Part model, mm, in its own coordinate system. Face numbers are marked on the shaded views. A direction names the side the tool comes from. Round coordinates to 2 decimals unless told otherwise and drop trailing zeros. Order: outer loops, then holes, each group sorted by start corner. A loop starts at its lowest first (then second) coordinate and runs counter-clockwise, first axis right, second up. Notation, with made-up numbers: (29, 3.25) - (71, 3.25) arc R15 cw to (71, 17.25) - close; hole circle Ø5 at (29.25, 74). An arc over 180 degrees is marked (long way). Return JSON: item names as keys, results as strings. Group by question number.
Item 1: Saw through at A-A on y = 0. List the corners of the cut face in (x, z).
Item 2: Tool access for the marked faces 1 and 2: list every direction of +Z, -Z, +X, -X, +Y, -Y with a clear straight run to the whole face (end or side of a thin tool).
Item 3: Saw through at C-C on y = -11. List the corners of the cut face in (x, z).
Item 4: Drop flat-ended pins along their axis: pin 1 (6 mm diameter, centred on y = 11.5, z = 130.5, fed in from -X); pin 2 (15 mm diameter, centred on x = -7, y = 0, fed in from +Z); pin 3 (3 mm diameter, centred on x = 91, z = 134.5, fed in from +Y). Give the stop position or say it passes through.
Item 5: Probe probe 1 along X at (y, z) = (-4.5, 82.5); probe 2 along Z at (x, y) = (7, 6); probe 3 along Z at (x, y) = (157, 3). List the from-to ranges inside material, lowest first.
Item 6: Saw through at B-B on y = 9. List the corners of the cut face in (x, z), and give its area (3 significant figures).
Item 7: Two-plate mould, pull along X, no slides. Class the marked faces 3 and 4: released by +X, released by -X, zero draft, split by the parting line, or undercut.
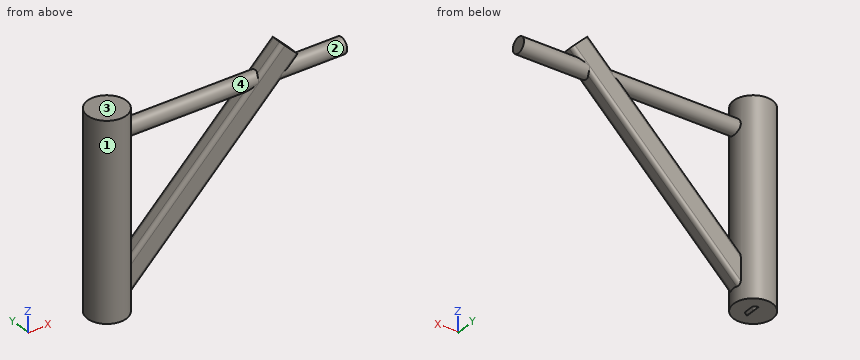
```python
from build123d import *

# Parameters (mm, degrees)
F0_R     = 15
F1_DEPTH = 150
F2_R     = 6
F3_DEPTH = 180
F7_DEPTH = 200


with BuildPart() as f1:
    # F0 (on Top) → F1 (new body)
    with BuildSketch(Plane.XY):
        Circle(F0_R)
    extrude(amount=F1_DEPTH)

    # F2 (on Right) → F3 (join)
    with BuildSketch(Plane.YZ):
        with Locations((0, 130.317822)):
            Circle(F2_R)
    extrude(amount=F3_DEPTH)

    # F6 (on face) → F7 (join)
    with BuildSketch(Plane(origin=(0, 0, 0), x_dir=(0.707107, 0, -0.707107), z_dir=(-0.707107, 0, -0.707107))):
        with BuildLine():
            Line((-0.517934, 6), (-12.829055, 6))
            ThreePointArc((-12.829055, 6), (-14.950375, 5.12132), (-15.829055, 3))
            Line((-15.829055, 3), (-15.829055, -3))
            ThreePointArc((-15.829055, -3), (-14.950375, -5.12132), (-12.829055, -6))
            Line((-12.829055, -6), (-0.517934, -6))
            ThreePointArc((-0.517934, -6), (1.603386, -5.12132), (2.482066, -3))
            Line((2.482066, -3), (2.482066, 3))
            ThreePointArc((2.482066, 3), (1.603386, 5.12132), (-0.517934, 6))
        make_face()
    extrude(amount=-F7_DEPTH)


solid = f1.part
```
Filled in:
{
 "1": {"outline": "(-15, 0) - (0, 0) - (1.76, -1.76) - (3.51, 0) - (15, 0) - (15, 11.49) - (127.83, 124.32) - (180, 124.32) - (180, 136.32) - (139.83, 136.32) - (143.18, 139.67) - (130.23, 152.61) - (113.93, 136.32) - (15, 136.32) - (15, 150) - (-15, 150) - close; hole (15, 37.39) - (101.93, 124.32) - (15, 124.32) - close"},
 "2": {"face 1": "none", "face 2": "+X"},
 "3": {"outline": "(-10.2, 0) - (10.2, 0) - (10.2, 150) - (-10.2, 150) - close"},
 "4": {"pin 1": "stops at x = -12.36", "pin 2": "stops at z = 150", "pin 3": "stops at y = 5.37"},
 "5": {"probe 1": "x = -14.31 to 14.31, 60.68 to 85.44", "probe 2": "z = 0 to 150", "probe 3": "z = 125.12 to 135.51"},
 "6": {"outline": "(-12, 0) - (12, 0) - (12, 150) - (-12, 150) - close", "area": "3,600 mm^2"},
 "7": {"face 3": "zero draft", "face 4": "undercut"}
}
